Geometry: final body of the model. Coordinates: model frame, mm. Face numbers are marked on the shaded views. A direction names the side the tool comes from. Give positions to 0.01 mm unless a question says otherwise; leave off trailing zeros. Write each loop counter-clockwise with the first axis right and the second up, starting at its lowest first coordinate (ties: lowest second). Pieces come first, ordered by that corner, then holes. Notation, with made-up numbers: (62.5, 47.5) -> (102.5, 47.5) arc R17 cw to (102.5, 77.5) -> close; hole circle Ø7 at (-20, -36.75). An arc over 180 degrees is marked (long way). Answer in a Markdown table with one row per item. Add a question column.
Item 1: Draft query along X for the marked faces 5, 6 and 7. Return one class per face: +X half, -X half, draft (parallel to the pull), parting line (faces both ways), or undercut.
Item 2: Material intervals for probe 1 along Y at (x, z) = (9.5, 3.5); probe 2 along Y at (x, z) = (0, 3.7); probe 3 along X at (y, z) = (-55.5, 3.65), sorted ascending. Write a range as from..to.
Item 3: Section query C-C on x = 0. Output: boundary loops of the cut face in (y, z).
Item 4: Section query B-B on z = 2.4. State how many separate pieces and enclosed holes the cut face has, plus the area to 3 significant figures.
Item 5: First-contact query: P1, Ø3, axis at y = -59, z = 4, coming from the +X side; P2, Ø1.6, axis at y = -23.5, z = 3.5, coming from the -X side; P3, Ø3, axis at x = 7.5, z = 3.5, coming from the +Y side. Flat tips, straight axial feed; report the tip coordinate or a pass-through.
Item 6: Section query A-A on y = -40.5. Output: boundary loops of the cut face in (x, z), plus the area to 3 significant figures.
Item 7: Section query D-D on x = -9.25. Output: boundary loops of the cut face in (y, z).
Item 8: Access query for the marked faces 1, 2, 3 and 4. Directions: +Z, -Z, +X, -X, +Y, -Y. A direction counts if a zero-diameter tool reaches every point of the face in a straight line with its end or side. Return the directions, or none.
```python
from build123d import *

# Parameters (mm, degrees)
EXTRUDE_1_DEPTH     = 5.5
SKETCH_3_R          = 1.05
SKETCH_3_W          = 12
SKETCH_3_H          = 22
CUT_EXTRUDE_2_DEPTH = 87.090069114
SKETCH_2_W          = 5.5
SKETCH_2_H          = 10
CUT_EXTRUDE_3_DEPTH = 87.090069114


with BuildPart() as part:
    # ｽｹｯﾁ1 → ﾎﾞｽ - 押し出し1 (new body)
    with BuildSketch(Plane.XY):
        with BuildLine():
            Line((-10, -19.595917942), (-10, -85))
            Line((-10, -85), (10, -85))
            Line((10, -85), (10, -19.595917942))
            ThreePointArc((10, -19.595917942), (10.503514163, -19.330705891), (11, -19.052558883))
            ThreePointArc((11, -19.052558883), (12.098076211, -14.954482672), (8, -13.856406461))
            ThreePointArc((8, -13.856406461), (0, -16), (-8, -13.856406461))
            ThreePointArc((-8, -13.856406461), (-12.098076211, -14.954482672), (-11, -19.052558883))
            ThreePointArc((-11, -19.052558883), (-10.503514163, -19.330705891), (-10, -19.595917942))
        make_face()
    extrude(amount=EXTRUDE_1_DEPTH)

    # ｽｹｯﾁ3 → ｶｯﾄ - 押し出し2 (cut, through all)
    with BuildSketch(Plane.XY.offset(5.5)):
        with Locations((0, -36.35)):
            Circle(SKETCH_3_R)
        with Locations((0, -63.65)):
            Circle(SKETCH_3_R)
        with Locations((0, -50)):
            Rectangle(SKETCH_3_W, SKETCH_3_H)
    extrude(amount=-CUT_EXTRUDE_2_DEPTH, mode=Mode.SUBTRACT)

    # ｽｹｯﾁ2 → ｶｯﾄ - 押し出し3 (cut, through all)
    with BuildSketch(Plane.XY.offset(5.5)):
        with Locations((-7.25, -75)):
            Rectangle(SKETCH_2_W, SKETCH_2_H)
        with Locations((-7.25, -30)):
            Rectangle(SKETCH_2_W, SKETCH_2_H)
        with Locations((7.25, -75)):
            Rectangle(SKETCH_2_W, SKETCH_2_H)
        with Locations((7.25, -30)):
            Rectangle(SKETCH_2_W, SKETCH_2_H)
    extrude(amount=-CUT_EXTRUDE_3_DEPTH, mode=Mode.SUBTRACT)


solid = part.part
```
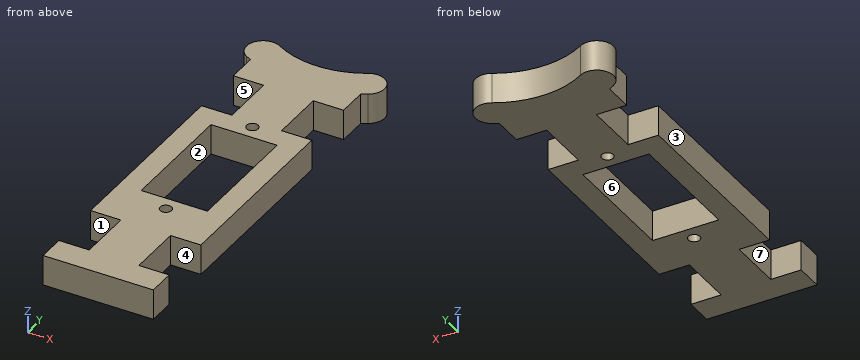
Findings below:
| question | item | result |
|---|---|---|
| 1 | face 5 | draft |
| 1 | face 6 | undercut |
| 1 | face 7 | -X half |
| 2 | probe 1 | y = -85..-80, -70..-35, -25..-13.45 |
| 2 | probe 2 | y = -85..-64.7, -62.6..-61, -39..-37.4, -35.3..-16 |
| 2 | probe 3 | x = -10..-6, 6..10 |
| 3 | outline | (-85, 0) -> (-64.7, 0) -> (-64.7, 5.5) -> (-85, 5.5) -> close; (-62.6, 0) -> (-61, 0) -> (-61, 5.5) -> (-62.6, 5.5) -> close; (-39, 0) -> (-37.4, 0) -> (-37.4, 5.5) -> (-39, 5.5) -> close; (-35.3, 0) -> (-16, 0) -> (-16, 5.5) -> (-35.3, 5.5) -> close |
| 4 | separate pieces | 1 |
| 4 | enclosed holes | 3 |
| 4 | area | 932 mm^2 |
| 5 | P1 | stops at x = 10 |
| 5 | P2 | stops at x = -10 |
| 5 | P3 | stops at y = -13.5 |
| 6 | outline | (-10, 0) -> (-6, 0) -> (-6, 5.5) -> (-10, 5.5) -> close; (6, 0) -> (10, 0) -> (10, 5.5) -> (6, 5.5) -> close |
| 6 | area | 44.0 mm^2 |
| 7 | outline | (-85, 0) -> (-80, 0) -> (-80, 5.5) -> (-85, 5.5) -> close; (-70, 0) -> (-35, 0) -> (-35, 5.5) -> (-70, 5.5) -> close; (-25, 0) -> (-13.46, 0) -> (-13.46, 5.5) -> (-25, 5.5) -> close |
| 8 | face 1 | +Z, -Z, -X |
| 8 | face 2 | +Z, -Z |
| 8 | face 3 | +Z, -Z, -X, -Y |
| 8 | face 4 | +Z, -Z, +X |
